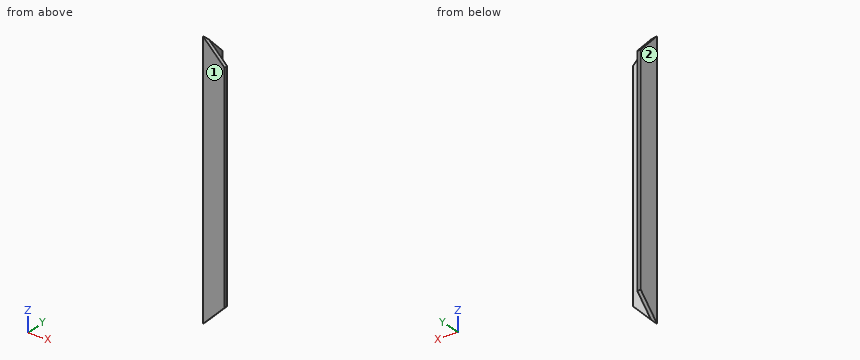
```python
from build123d import *

# Parameters (mm, degrees)
F1_DEPTH = 600
F3_DEPTH = 8
F5_DEPTH = 8
F7_DEPTH = 8
F9_DEPTH = 8


with BuildPart() as f1:
    # F0 (on Top) → F1 (new body)
    with BuildSketch(Plane.XY):
        Polygon((0, 50), (0, 0), (50, 0), (50, 8), (8, 8), (8, 50), align=None)
    extrude(amount=F1_DEPTH)

    # F2 (on face) → F3 (cut, through all)
    with BuildSketch(Plane.XZ):
        Polygon((50, 600), (0, 600), (50, 550), align=None)
    extrude(amount=-F3_DEPTH, mode=Mode.SUBTRACT)

    # F4 (on face) → F5 (cut, through all)
    with BuildSketch(Plane(origin=(0, 0, 0), x_dir=(0, -1, 0), z_dir=(-1, 0, 0))):
        Polygon((-50, 550), (0, 600), (-8, 600), (-50, 600), align=None)
    extrude(amount=-F5_DEPTH, mode=Mode.SUBTRACT)

    # F6 (on face) → F7 (cut, through all)
    with BuildSketch(Plane.XZ):
        Polygon((50, 50), (0, 0), (50, 0), align=None)
    extrude(amount=-F7_DEPTH, mode=Mode.SUBTRACT)

    # F8 (on face) → F9 (cut, through all)
    with BuildSketch(Plane(origin=(0, 0, 0), x_dir=(0, -1, 0), z_dir=(-1, 0, 0))):
        Polygon((-8, 0), (0, 0), (-50, 50), (-50, 0), align=None)
    extrude(amount=-F9_DEPTH, mode=Mode.SUBTRACT)


solid = f1.part
```
Part model, mm, in its own coordinate system. Face numbers are marked on the shaded views. Round coordinates to 2 decimals unless told otherwise and drop trailing zeros. Loops run counter-clockwise (first coordinate to the right, second up) from the corner with the lowest first, then second, coordinate; pieces in that order, holes last.
1. Two-plate mould, pull along Y, no slides. Class the marked faces 1 and 2: pulls with the +Y half, pulls with the -Y half, needs draft (parallel to the pull), parting line crosses it, or undercut.
Solutions:
face 1: pulls with the -Y half
face 2: needs draft
2. Slice it at B-B (x = 18.5). Give the cut face in (y, z), and give its area (3 significant figures).
Solutions:
outline: (0, 18.5) - (8, 18.5) - (8, 581.5) - (0, 581.5) - close
area: 4,500 mm2
3. Slice it at A-A (z = 268.5). Give the cut face in (x, y).
Solutions:
outline: (0, 0) - (50, 0) - (50, 8) - (8, 8) - (8, 50) - (0, 50) - close
4. Flat gauge pins, fed straight in: pin 1 (1 mm diameter, centred on x = 13.5, z = 70, fed in from +Y); pin 2 (6 mm diameter, centred on x = 8, y = 43.5, fed in from +Z). Where does each tip first touch, or does it go through?
Solutions:
pin 1: stops at y = 8
pin 2: stops at z = 559.5
5. Drill centre lines: line 1 along Y through (x, z) = (46.5, 69); line 2 along Z through (x, y) = (34, 7). Where is each one in solid material? Low to high.
Solutions:
line 1: y = 0 to 8
line 2: z = 34 to 566
6. Slice it at C-C (y = 13). Give the cut face in (x, z).
Solutions:
outline: (0, 13) - (8, 13) - (8, 587) - (0, 587) - close
